Input: dimensioned drawing with shaded views. Units: mm. Origin: part minimum x, y, z. A direction names the side the tool comes from. Round coordinates to 2 decimals unless told otherwise and drop trailing zeros. Loops run counter-clockwise (first coordinate to the right, second up) from the corner with the lowest first, then second, coordinate; pieces in that order, holes last. Notation, with made-up numbers: (54.25, 53) -> (93.25, 53) arc R34 cw to (93.25, 91) -> close; hole circle Ø10 at (45.25, 44.25). An arc over 180 degrees is marked (long way). Answer as a JSON object with one key per item and string values.
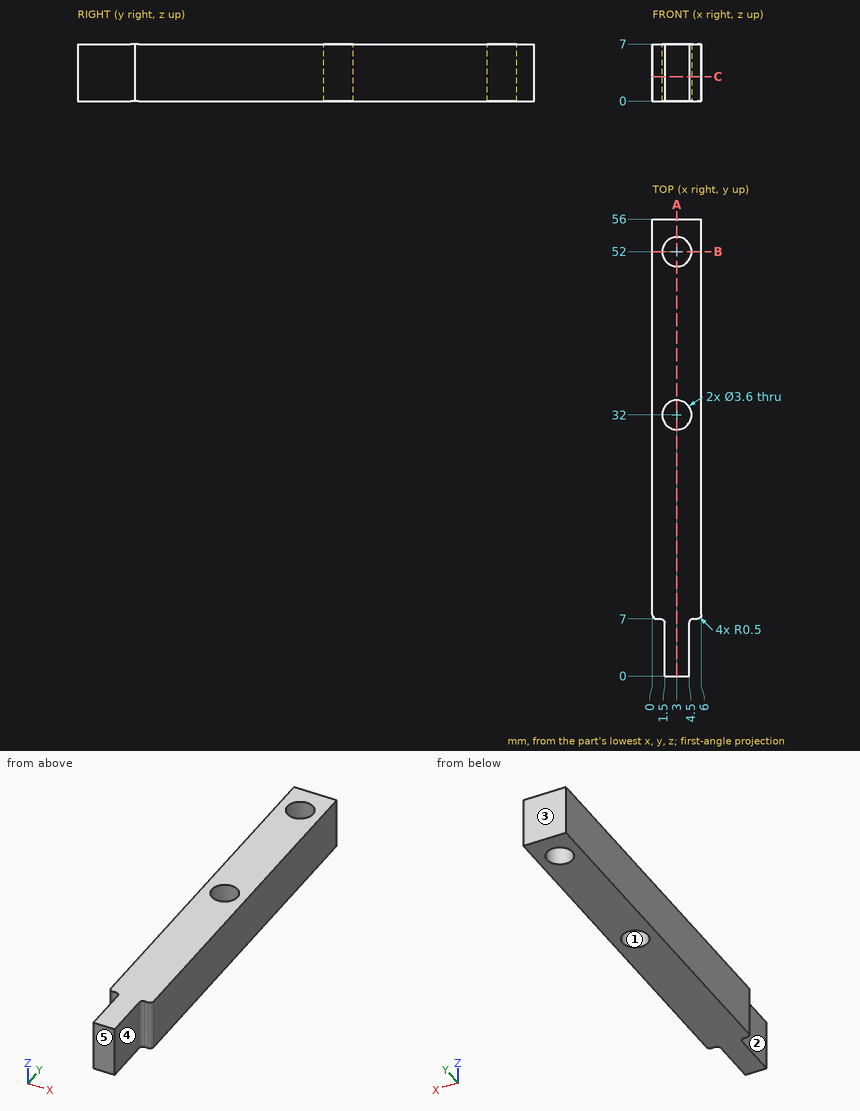
1) Section A-A, the plane x = 3. Output: boundary loops of the cut face in (y, z).
Output:
{"outline": "(0, 0) -> (30.2, 0) -> (30.2, 7) -> (0, 7) -> close; (33.8, 0) -> (50.2, 0) -> (50.2, 7) -> (33.8, 7) -> close; (53.8, 0) -> (56, 0) -> (56, 7) -> (53.8, 7) -> close"}
2) Draft query along X for the marked faces 1, 2 and 3. Return one class per face: +X half, -X half, draft (parallel to the pull), parting line (faces both ways), or undercut.
Output:
{"face 1": "undercut", "face 2": "-X half", "face 3": "draft"}
3) Section B-B, the plane y = 52. Output: boundary loops of the cut face in (x, z), plus the area to 3 significant figures.
Output:
{"outline": "(0, 0) -> (1.2, 0) -> (1.2, 7) -> (0, 7) -> close; (4.8, 0) -> (6, 0) -> (6, 7) -> (4.8, 7) -> close", "area": "16.8 mm^2"}
4) Reachability of the marked faces 4 and 5 from +Z, -Z, +X, -X, +Y, -Y: full face, straight path, thin tool, end or side. Return the list, or none.
Output:
{"face 4": "+Z, -Z, +X, -Y", "face 5": "+Z, -Z, +X, -X, -Y"}
5) Ray query, probe 1 along Y at (x, z) = (3, 5.75); probe 2 along Y at (x, z) = (4.1, 3.25); probe 3 along X at (y, z) = (53, 1.5). Return the intervals inside material, ascending.
Output:
{"probe 1": "y = 0 to 30.2, 33.8 to 50.2, 53.8 to 56", "probe 2": "y = 0 to 30.58, 33.42 to 50.58, 53.42 to 56", "probe 3": "x = 0 to 1.5, 4.5 to 6"}
6) Contact query for a flat-ended pin moving along its axis: P1, Ø0.6, axis at x = 5, z = 5, coming from the -Y side. Output: stop coordinate, or through.
Output:
{"P1": "stops at y = 6.9"}
7) Section C-C, the plane z = 3. Output: boundary loops of the cut face in (x, y), plus the area to 3 significant figures.
Output:
{"outline": "(0, 7.5) arc R0.5 ccw to (0.5, 7) -> (1, 7) arc R0.5 cw to (1.5, 6.5) -> (1.5, 0) -> (4.5, 0) -> (4.5, 6.5) arc R0.5 cw to (5, 7) -> (5.5, 7) arc R0.5 ccw to (6, 7.5) -> (6, 56) -> (0, 56) -> close; hole circle Ø3.6 at (3, 32); hole circle Ø3.6 at (3, 52)", "area": "295 mm^2"}
